```python
from build123d import *

# Parameters (mm, degrees)
F0_R     = 5
F1_DEPTH = 15
F2_DEPTH = 20
F4_DEPTH = 30.001


with BuildPart() as f1:
    # F0 (on Top) → F1 (new body)
    with BuildSketch(Plane.XY):
        with BuildLine():
            ThreePointArc((0, -10), (10, 0), (0, 10))
            ThreePointArc((0, 10), (-10, 0), (0, -10))
        make_face()
        Circle(F0_R, mode=Mode.SUBTRACT)
        with BuildLine():
            Line((15, 10), (0, 10))
            ThreePointArc((0, 10), (10, 0), (0, -10))
            Line((0, -10), (15, -10))
            Line((15, -10), (20, -5))
            Line((20, -5), (20, 5))
            Line((20, 5), (15, 10))
        make_face()
    extrude(amount=F1_DEPTH)

    # F0 (on Top) → F2 (join)
    with BuildSketch(Plane.XY):
        with BuildLine():
            ThreePointArc((0, -10), (10, 0), (0, 10))
            ThreePointArc((0, 10), (-10, 0), (0, -10))
        make_face()
        Circle(F0_R, mode=Mode.SUBTRACT)
    extrude(amount=F2_DEPTH)

    # F3 (on face) → F4 (cut, through all)
    with BuildSketch(Plane.YZ.offset(20)):
        Polygon((2.5, 10), (2.5, 15), (2.5, 20), (-2.5, 20), (-2.5, 15), (-2.5, 10), align=None)
    extrude(amount=-F4_DEPTH, mode=Mode.SUBTRACT)


solid = f1.part
```
Check sheet for the modelled part. Datum: model origin and axes. Units: mm. A direction names the side the tool comes from. Round coordinates to 2 decimals unless told otherwise and drop trailing zeros. Loops run counter-clockwise (first coordinate to the right, second up) from the corner with the lowest first, then second, coordinate; pieces in that order, holes last. Notation, with made-up numbers: (-16.75, 73.5) -> (-6.75, 73.5) arc R24 ccw to (-6.75, 101.5) -> close; hole circle Ø5 at (-31, 51.25). An arc over 180 degrees is marked (long way). Answer in a Markdown table with one row per item.
Q1. Sectioned sample at D-D on z = 2.25. Enter the section's corners in (x, y).
Data:
| item | result |
|---|---|
| outline | (0, -10) -> (15, -10) -> (20, -5) -> (20, 5) -> (15, 10) -> (0, 10) arc R10 ccw to start; hole circle Ø10 at (0, 0) |
Q2. Thickness scan on L1, parallel to Y at x = 0.25, z = 18; L2, parallel to X at y = 0, z = 8.75; L3, parallel to Y at x = -2.5, z = 11.25. Record the ranges inside material, lowest first.
Data:
| item | result |
|---|---|
| L1 | y = -10 to -4.99, 4.99 to 10 |
| L2 | x = -10 to -5, 5 to 20 |
| L3 | y = -9.68 to -4.33, 4.33 to 9.68 |
Q3. Sectioned sample at B-B on z = 12. Enter the section's corners in (x, y).
Data:
| item | result |
|---|---|
| outline | (-9.68, -2.5) arc R10 ccw to (0, -10) -> (15, -10) -> (20, -5) -> (20, -2.5) -> (4.33, -2.5) arc R5 cw to (-4.33, -2.5) -> close; (-9.68, 2.5) -> (-4.33, 2.5) arc R5 cw to (4.33, 2.5) -> (20, 2.5) -> (20, 5) -> (15, 10) -> (0, 10) arc R10 ccw to start |
Q4. Sectioned sample at C-C on x = 3. Enter the section's corners in (y, z).
Data:
| item | result |
|---|---|
| outline | (-10, 0) -> (-4, 0) -> (-4, 20) -> (-9.54, 20) -> (-9.54, 15) -> (-10, 15) -> close; (4, 0) -> (10, 0) -> (10, 15) -> (9.54, 15) -> (9.54, 20) -> (4, 20) -> close |
Q5. Sectioned sample at A-A on y = 0. Enter the section's corners in (x, z), then the cut area to 3 significant figures.
Data:
| item | result |
|---|---|
| outline | (-10, 0) -> (-5, 0) -> (-5, 10) -> (-10, 10) -> close; (5, 0) -> (20, 0) -> (20, 10) -> (5, 10) -> close |
| area | 200 mm^2 |
Q6. Release check for a two-part mould opening along Y. For faces 4 (the face through (-7, 2.5, 15)), 5 (the face through (18, 7, 7)), 6 (the face through (20, 0, 6)) record: released by +Y, released by -Y, zero draft, split by the parting line, or undercut.
Data:
| item | result |
|---|---|
| face 4 | undercut |
| face 5 | released by +Y |
| face 6 | zero draft |
Q7. Set-up check for faces 1 (the face through (-10, 0, 8)), 2 (the face through (-7, 0, 10)), 3 (the face through (12, -6, 15)): record each of +Z, -Z, +X, -X, +Y, -Y from which the full face is reachable in a straight line by a thin tool's end or side.
Data:
| item | result |
|---|---|
| face 1 | +Z |
| face 2 | +Z, +X, -X |
| face 3 | +Z, +X, -Y |
Q8. Go/stop test with flat-tipped pins: P1, Ø8, axis at x = 14, y = 2.5, coming from the +Z side; P2, Ø4.5, axis at x = -7.5, z = 15.5, coming from the +Y side; P3, Ø6, axis at x = -6.5, z = 15.5, coming from the -Y side. Record where each tip stops, or that it passes through.
Data:
| item | result |
|---|---|
| P1 | stops at z = 15 |
| P2 | stops at y = 8.51 |
| P3 | stops at y = -9.37 |
